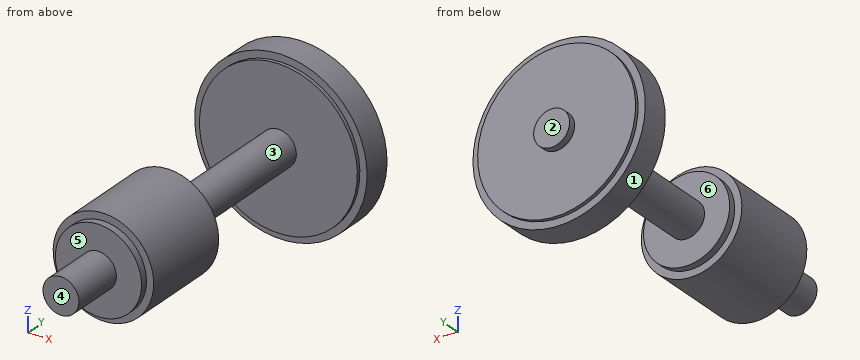
```python
from build123d import *

# Parameters (mm, degrees)
F2_W = 0.2
F2_H = 0.2
F4_W = 0.1
F4_H = 0.2


with BuildPart() as f1:
    # F0 (on Right) → F1 (revolve)
    with BuildSketch(Plane.YZ):
        Polygon((-1.5, 0.5), (-1.5, 0), (8.4, 0), (8.4, 0.5), (8.2, 0.5), (8.2, 2.4), (7.2, 2.4), (7.2, 0.5), (3, 0.5), (3, 1.4), (0, 1.4), (0, 0.5), align=None)
    revolve(axis=Axis((0, 3.45, 0), (0, -1, 0)))

    # F2 (on Right) → F3 (revolve, cut)
    with BuildSketch(Plane.YZ):
        with Locations((2.9, 1.3)):
            Rectangle(F2_W, F2_H)
        with Locations((0.1, 1.3)):
            Rectangle(F2_W, F2_H)
    revolve(axis=Axis((0, 3.45, 0), (0, -1, 0)), mode=Mode.SUBTRACT)

    # F4 (on Right) → F5 (revolve, cut)
    with BuildSketch(Plane.YZ):
        with Locations((8.15, 2.3)):
            Rectangle(F4_W, F4_H)
        with Locations((7.25, 2.3)):
            Rectangle(F4_W, F4_H)
    revolve(axis=Axis((0, 3.45, 0), (0, -1, 0)), mode=Mode.SUBTRACT)


solid = f1.part
```
Geometry: final body of the model. Coordinates: model frame, mm. Face numbers are marked on the shaded views. A direction names the side the tool comes from. Round coordinates to 2 decimals unless told otherwise and drop trailing zeros. Order: outer loops, then holes, each group sorted by start corner. A loop starts at its lowest first (then second) coordinate and runs counter-clockwise, first axis right, second up. Notation, with made-up numbers: (43, 58) -> (71, 58) arc R25 cw to (71, 93) -> close; hole circle Ø8 at (-32.5, 66.5). An arc over 180 degrees is marked (long way). Use one line per item in the form item = value.
(1) Access query for the marked faces 4, 5 and 6. Directions: +Z, -Z, +X, -X, +Y, -Y. A direction counts if a zero-diameter tool reaches every point of the face in a straight line with its end or side. Return the directions, or none.
Results list:
face_4 = +Z, -Z, +X, -X, -Y
face_5 = -Y
face_6 = none
(2) Section C-C on z = 1.85. Return loops of the section in (x, y).
Results list:
outline = (-1.53, 7.3) -> (-1.19, 7.3) -> (-1.19, 7.2) -> (1.19, 7.2) -> (1.19, 7.3) -> (1.53, 7.3) -> (1.53, 8.1) -> (1.19, 8.1) -> (1.19, 8.2) -> (-1.19, 8.2) -> (-1.19, 8.1) -> (-1.53, 8.1) -> close
(3) Section D-D on y = 4.25. Return loops of the section in (x, z).
Results list:
outline = circle Ø1 at (0, 0)
(4) Section B-B on x = 1.9. Return loops of the section in (y, z), and give its area (3 significant figures).
Results list:
outline = (7.2, -1.11) -> (7.3, -1.11) -> (7.3, -1.47) -> (8.1, -1.47) -> (8.1, -1.11) -> (8.2, -1.11) -> (8.2, 1.11) -> (8.1, 1.11) -> (8.1, 1.47) -> (7.3, 1.47) -> (7.3, 1.11) -> (7.2, 1.11) -> close
area = 2.79 mm^2
(5) Ray query, probe 1 along Y at (x, z) = (-1.25, 0); probe 2 along X at (y, z) = (4, 0); probe 3 along Y at (x, z) = (0.3, 1.4). Return the intervals inside material, ascending. Write a range as [from, to].
Results list:
probe_1 = [0.2, 2.8], [7.2, 8.2]
probe_2 = [-0.5, 0.5]
probe_3 = [7.2, 8.2]
(6) Draft query along Y for the marked faces 1, 2 and 3. Return one class per face: pulls with the +Y half, pulls with the -Y half, needs draft (parallel to the pull), parting line crosses it, or undercut.
Results list:
face_1 = needs draft
face_2 = pulls with the +Y half
face_3 = undercut
(7) Section A-A on z = -1.05. Return loops of the section in (x, y), and give its area (3 significant figures).
Results list:
outline = (-2.16, 7.3) -> (-1.93, 7.3) -> (-1.93, 7.2) -> (1.93, 7.2) -> (1.93, 7.3) -> (2.16, 7.3) -> (2.16, 8.1) -> (1.93, 8.1) -> (1.93, 8.2) -> (-1.93, 8.2) -> (-1.93, 8.1) -> (-2.16, 8.1) -> close; (-0.93, 0.2) -> (-0.58, 0.2) -> (-0.58, 0) -> (0.58, 0) -> (0.58, 0.2) -> (0.93, 0.2) -> (0.93, 2.8) -> (0.58, 2.8) -> (0.58, 3) -> (-0.58, 3) -> (-0.58, 2.8) -> (-0.93, 2.8) -> close
area = 9.51 mm^2
